Geometry check sheet. Reference: the model listing, model coordinates, mm. Face numbers are marked on the shaded views. A direction names the side the tool comes from. Round coordinates to 2 decimals unless told otherwise and drop trailing zeros. Write each loop counter-clockwise with the first axis right and the second up, starting at its lowest first coordinate (ties: lowest second). Pieces come first, ordered by that corner, then holes. Notation, with made-up numbers: (67.5, -19) - (89.5, -19) arc R30 cw to (89.5, 9) - close; hole circle Ø2 at (19, 18.5). An arc over 180 degrees is marked (long way). Return JSON: item names as keys, results as strings.
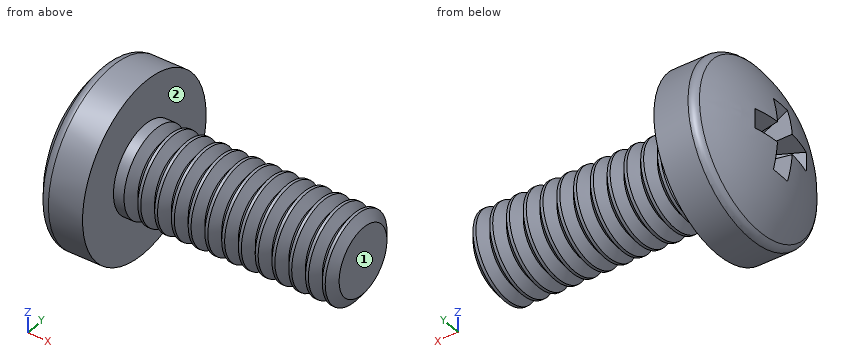
```python
from build123d import *

# Parameters (mm, degrees)
SKETCH3_W         = 0.48
SKETCH3_H         = 1.82
SKETCH4_W         = 0.24
SKETCH4_H         = 0.24
CIRPATTERN1_COUNT = 2
CIRPATTERN1_ANGLE = 90
THDSCHPAT_COUNT   = 13
THDSCHPAT_PITCH   = 0.383333333


with BuildPart() as part:
    # BodySke → Base-Revolve (revolve)
    with BuildSketch(Plane.XY):
        with BuildLine():
            Line((1.6, 1), (1.6, 2))
            Line((1.6, 2), (0.820084035, 2))
            ThreePointArc((0.820084035, 2), (0.712029995, 1.974299613), (0.627117876, 1.902702703))
            ThreePointArc((0.627117876, 1.902702703), (0.160820604, 1.001692868), (0, 0))
            Line((0, 0), (6.6, 0))
            Line((6.6, 0), (6.6, 1))
            Line((6.6, 1), (1.6, 1))
        make_face()
    revolve(axis=Axis((-25.4, 0, 0), (1, 0, 0)))

    # Sketch3 → Cut-Loft1 section 0
    with BuildSketch(Plane(origin=(0, 0, 0), x_dir=(0, 0, -1), z_dir=(1, 0, 0))):
        Rectangle(SKETCH3_W, SKETCH3_H)
    # Sketch4 → Cut-Loft1 section 1
    with BuildSketch(Plane(origin=(1.19, 0, 0), x_dir=(0, 0, -1), z_dir=(1, 0, 0))):
        Rectangle(SKETCH4_W, SKETCH4_H)
    cut_loft1 = loft(mode=Mode.SUBTRACT)

    # CirPattern1: Cut-Loft1 ×2 about axis
    cirpattern1_axis = Axis((0, 0, 0), (1, 0, 0))
    for i in range(1, CIRPATTERN1_COUNT):
        add(cut_loft1.rotate(cirpattern1_axis, i * CIRPATTERN1_ANGLE / (CIRPATTERN1_COUNT - 1)), mode=Mode.SUBTRACT)

    # ThdSchSke → ThreadSchematic (revolve, cut)
    with BuildSketch(Plane.XY):
        Polygon((2, -0.774), (1.841753096, -1), (1.841753096, -1.25), (2.158246904, -1.25), (2.158246904, -1), align=None)
    threadschematic = revolve(axis=Axis((-3.175, 0, 0), (1, 0, 0)), mode=Mode.SUBTRACT)

    # ThdSchPat: ThreadSchematic ×13
    with Locations(*[(i * THDSCHPAT_PITCH, 0, 0) for i in range(1, THDSCHPAT_COUNT)]):
        add(threadschematic, mode=Mode.SUBTRACT)


solid = part.part
```
(1) Access from +Z, -Z, +X, -X, +Y, -Y to the whole of each face (thin tool, end or side, straight path). Record for the marked faces 1 and 2.
Response values:
{"face 1": "+Z, -Z, +X, +Y, -Y", "face 2": "+X"}
(2) Material ranges on line 1 along Y through (x, z) = (1, -0.1); line 2 along X through (y, z) = (-0.6, -1.4); line 3 along Y through (x, z) = (3.5, -0.5), recorded low to high. Write a range as [from, to].
Response values:
{"line 1": "y = [-2, -0.25], [0.25, 2]", "line 2": "x = [0.39, 1.6]", "line 3": "y = [-0.65, 0.65]"}
(3) Section check A-A, the plane x = 4. Enter the section's corners in (y, z), plus the area to 3 significant figures.
Response values:
{"outline": "circle Ø1.79 at (0, 0)", "area": "2.51 mm^2"}
(4) Gauge pin test, flat ends, axial feed: pin 1 (1 mm diameter, centred on x = 2, z = -1, fed in from +Y); pin 2 (2 mm diameter, centred on x = 1.5, y = 0.5, fed in from -Z). Record the tip position at first contact, or that the pin passes through.
Response values:
{"pin 1": "stops at y = 1.87", "pin 2": "stops at z = -2"}
